```python
from build123d import *

# Parameters (mm, degrees)
F0_W     = 4.155186
F0_H     = 29.55925
F6_R     = 8.4455
F7_DEPTH = 4.22275


with BuildPart() as f3:
    # F0 (on Right) → F3 (revolve)
    with BuildSketch(Plane.YZ):
        with Locations((-2.077593, 0)):
            Rectangle(F0_W, F0_H)
    revolve(axis=Axis((0, 0, 0), (0, 0, -1)))

    # F1 (on Right) → F4 (revolve)
    with BuildSketch(Plane.YZ):
        Polygon((-12.7995307084, -7.3898125), (12.7995307084, 7.3898125), (10.7219377084, 10.9883091334), (-14.8771237084, -3.7913158666), align=None)
    revolve(axis=Axis((0, 0, 0), (0, -0.8660254038, -0.5)))

    # F2 (on Right) → F5 (revolve)
    with BuildSketch(Plane.YZ):
        Polygon((-12.7995307084, 7.3898125), (12.7995307084, -7.3898125), (14.8771237084, -3.7913158666), (-10.7219377084, 10.9883091334), align=None)
    revolve(axis=Axis((0, 0, 0), (0, -0.8660254038, 0.5)))

    # F6 (on Right) → F7 (join, symmetric)
    with BuildSketch(Plane.YZ):
        Circle(F6_R)
    extrude(amount=F7_DEPTH, both=True)


solid = f3.part
```
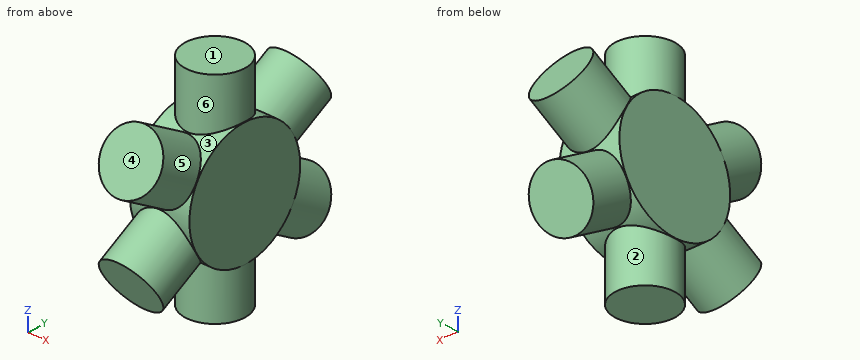
Build history of the part. All positions in model axes, mm. Face numbers are marked on the shaded views. A direction names the side the tool comes from. Round coordinates to 2 decimals unless told otherwise and drop trailing zeros. Write each loop counter-clockwise with the first axis right and the second up, starting at its lowest first coordinate (ties: lowest second). Pieces come first, ordered by that corner, then holes.
1) Pin check, flat tips, straight feed: pin 1 (2 mm diameter, centred on x = 1, z = 9, fed in from -Y); pin 2 (1 mm diameter, centred on x = -2, z = 10.5, fed in from +Y); pin 3 (1.5 mm diameter, centred on x = -1.5, z = -4, fed in from -Y). Stop position of each tip, or through.
2) Band-saw the part on A-A, the plane y = 2.5. List the corners of the cut face in (x, z).
3) Mould opens along Z. For the marked faces 4, 5 and 6 say: +Z half, -Z half, draft (parallel to the pull), parting line (faces both ways), or undercut.
4) Drill centre lines: probe 1 along Y at (x, z) = (-2.5, -8.5); probe 2 along Z at (x, y) = (-2.5, -11); probe 3 along Z at (x, y) = (-1.5, -12.25). Where is each one in solid material? Low to high.
5) 3-axis set-ups, long thin cutter, end or side, ignore diameter. For the marked faces 1, 2 and 3: which of +Z, -Z, +X, -X, +Y, -Y reach the whole face in a straight line?
6) Band-saw the part on C-C, the plane x = -3. List the corners of the cut face in (y, z) (1 decimal), and give its area (3 significant figures).
Ans:
1. pin 1: stops at y = -12.45
1. pin 2: stops at y = 11.29
1. pin 3: stops at y = -14.84
2. outline: (-4.22, -8.07) - (-3.32, -8.07) - (-3.32, -14.78) - (3.32, -14.78) - (3.32, -8.07) - (4.22, -8.07) - (4.22, 8.07) - (3.32, 8.07) - (3.32, 14.78) - (-3.32, 14.78) - (-3.32, 8.07) - (-4.22, 8.07) - close
3. face 4: +Z half
3. face 5: undercut
3. face 6: draft
4. probe 1: y = -12.16 to -8.08, -3.32 to 3.32, 8.08 to 12.16
4. probe 2: z = -10.18 to -2.52, 2.52 to 10.18
4. probe 3: z = -8.34 to -2.6, 2.6 to 8.34
5. face 1: +Z, +X, -X, +Y, -Y
5. face 2: -Z
5. face 3: none
6. outline: (-14.2, -4.9) - (-11.4, -9.9) - (-5.4, -6.5) arc R8.4 ccw to (-2.9, -7.9) - (-2.9, -14.8) - (2.9, -14.8) - (2.9, -7.9) arc R8.4 ccw to (5.4, -6.5) - (11.4, -9.9) - (14.2, -4.9) - (8.3, -1.5) arc R8.4 ccw to (8.3, 1.5) - (14.2, 4.9) - (11.4, 9.9) - (5.4, 6.5) arc R8.4 ccw to (2.9, 7.9) - (2.9, 14.8) - (-2.9, 14.8) - (-2.9, 7.9) arc R8.4 ccw to (-5.4, 6.5) - (-11.4, 9.9) - (-14.2, 4.9) - (-8.3, 1.5) arc R8.4 ccw to (-8.3, -1.5) - close
6. area: 448 mm2
